The drawing under review shows one solid part. Ordinate dimensions are in mm from its lowest x, y, z. A direction names the side the tool comes from. Give positions to 0.01 mm unless a question says otherwise; leave off trailing zeros. Write each loop counter-clockwise with the first axis right and the second up, starting at its lowest first coordinate (ties: lowest second). Pieces come first, ordered by that corner, then holes.
Q1. We need section A-A (x = 17.5). Write out the cut boundary in (y, z).
Q2. Machinability: for the marked faces 1 and 2, which of the approach directions +Z, -Z, +X, -X, +Y, -Y give a long, thin tool a straight path to every point of the face, cutting with its end or side? Answer none if there is none.
Q3. We need section B-B (z = 16.25). Write out the cut boundary in (x, y), then the cut area to 3 significant figures.
Q4. We need section C-C (y = 2.4). Write out the cut boundary in (x, z), then the cut area to 3 significant figures.
Q5. We need section D-D (x = 10.5). Write out the cut boundary in (y, z), then the cut area to 3 significant figures.
Q6. For line 1 (Z direction, x = 17.5, y = 1.35); line 2 (X direction, y = 2.4, z = 21.5); line 3 (X direction, y = 1.8, z = 11.25), list the stretches that pass through material, from the lowest coordinate up.
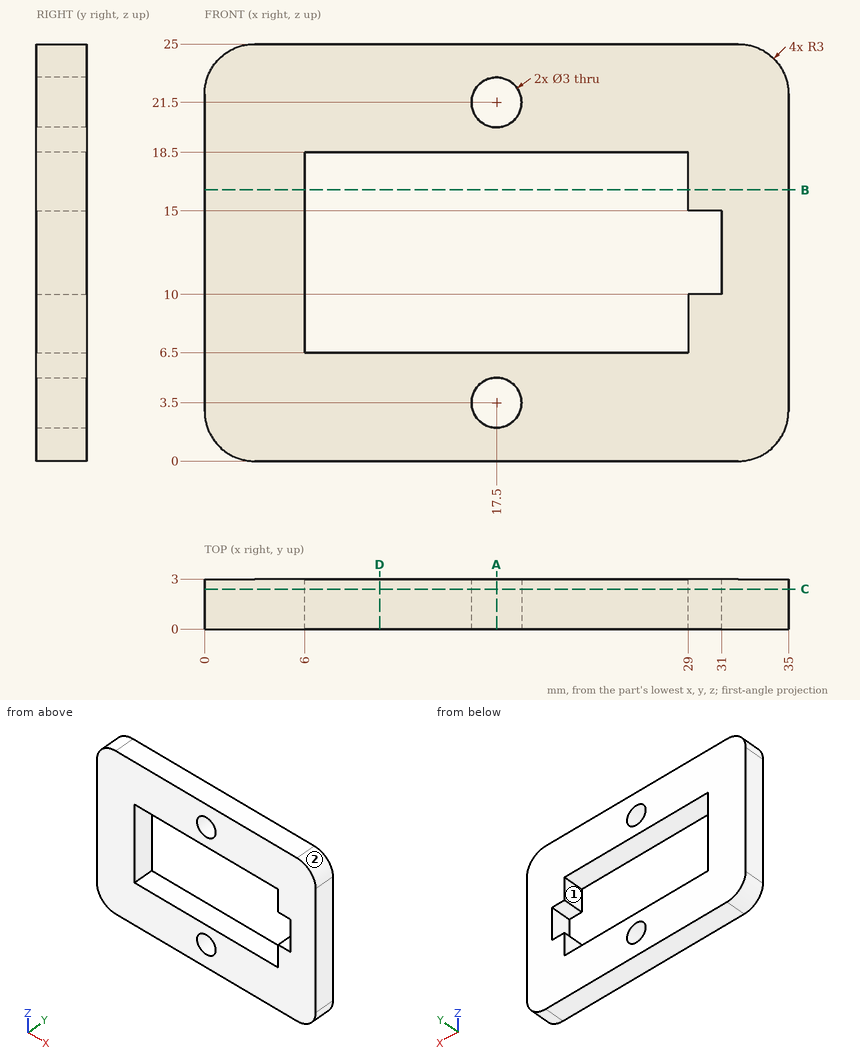
Computed:
1. outline: (0, 0) - (3, 0) - (3, 2) - (0, 2) - close; (0, 5) - (3, 5) - (3, 6.5) - (0, 6.5) - close; (0, 18.5) - (3, 18.5) - (3, 20) - (0, 20) - close; (0, 23) - (3, 23) - (3, 25) - (0, 25) - close
2. face 1: +Y, -Y
2. face 2: +Z, +X, +Y, -Y
3. outline: (0, 0) - (6, 0) - (6, 3) - (0, 3) - close; (29, 0) - (35, 0) - (35, 3) - (29, 3) - close
3. area: 36.0 mm2
4. outline: (0, 3) arc R3 ccw to (3, 0) - (32, 0) arc R3 ccw to (35, 3) - (35, 22) arc R3 ccw to (32, 25) - (3, 25) arc R3 ccw to (0, 22) - close; hole (6, 6.5) - (29, 6.5) - (29, 10) - (31, 10) - (31, 15) - (29, 15) - (29, 18.5) - (6, 18.5) - close; hole circle Ø3 at (17.5, 3.5); hole circle Ø3 at (17.5, 21.5)
4. area: 567 mm2
5. outline: (0, 0) - (3, 0) - (3, 6.5) - (0, 6.5) - close; (0, 18.5) - (3, 18.5) - (3, 25) - (0, 25) - close
5. area: 39.0 mm2
6. line 1: z = 0 to 2, 5 to 6.5, 18.5 to 20, 23 to 25
6. line 2: x = 0 to 16, 19 to 35
6. line 3: x = 0 to 6, 31 to 35
